Geometry: final body of the model. Coordinates: model frame, mm. A direction names the side the tool comes from. Round coordinates to 2 decimals unless told otherwise and drop trailing zeros. Loops run counter-clockwise (first coordinate to the right, second up) from the corner with the lowest first, then second, coordinate; pieces in that order, holes last. Notation, with made-up numbers: (38, 5.25) -> (75, 5.25) arc R28 ccw to (75, 31.25) -> close; hole circle Ø1 at (37.25, 17.5). An arc over 180 degrees is marked (long way). Answer in a Markdown table with one row per item.
```python
from build123d import *

# Parameters (mm, degrees)
SKETCH1_R           = 2.75
BOSS_EXTRUDE1_DEPTH = 12
SKETCH2_W           = 16
SKETCH2_H           = 46.496113018
CUT_EXTRUDE1_DEPTH  = 229.638147517
SKETCH3_R           = 2.1
CUT_EXTRUDE2_DEPTH  = 229.638147517
CUT_EXTRUDE3_DEPTH  = 229.638147517
FILLET1_R           = 3
FILLET2_R           = 2
SKETCH6_R           = 1.8
CUT_EXTRUDE4_DEPTH  = 229.638147652
CHAMFER1_SIZE       = 1.678199262
CHAMFER1_SIZE_2     = 2


with BuildPart() as part:
    # Sketch1 → Boss-Extrude1 (new body)
    with BuildSketch(Plane(origin=(0, 0, 0), x_dir=(1, 0, 0), z_dir=(0, 1, 0))):
        with BuildLine():
            Line((0, 71.75), (68.4, 71.75))
            Line((68.4, 71.75), (74.4, 82.75))
            Line((74.4, 82.75), (119.4, 82.75))
            Line((119.4, 82.75), (125.4, 71.75))
            Line((125.4, 71.75), (212.8, 71.75))
            Line((212.8, 71.75), (212.8, 43.975))
            Line((212.8, 43.975), (202.281088693, 43.975))
            ThreePointArc((202.281088693, 43.975), (201.490544346, 44.652363805), (200.7, 43.975))
            Line((200.7, 43.975), (200.7, 27.775))
            ThreePointArc((200.7, 27.775), (201.490544346, 27.097636195), (202.281088693, 27.775))
            Line((202.281088693, 27.775), (212.8, 27.775))
            Line((212.8, 27.775), (212.8, 0))
            Line((212.8, 0), (106.4, 0))
            Line((106.4, 0), (0, 0))
            Line((0, 0), (0, 27.775))
            Line((0, 27.775), (10.518911307, 27.775))
            ThreePointArc((10.518911307, 27.775), (11.309455654, 27.097636195), (12.1, 27.775))
            Line((12.1, 27.775), (12.1, 43.975))
            ThreePointArc((12.1, 43.975), (11.309455654, 44.652363805), (10.518911307, 43.975))
            Line((10.518911307, 43.975), (0, 43.975))
            Line((0, 43.975), (0, 71.75))
        make_face()
        with Locations(Location((39, 59.75, 0), (0, 0, 270))):
            Circle(SKETCH1_R, mode=Mode.SUBTRACT)
        with Locations(Location((39, 12, 0), (0, 0, 270))):
            Circle(SKETCH1_R, mode=Mode.SUBTRACT)
        with Locations(Location((173.8, 59.75, 0), (0, 0, 90))):
            Circle(SKETCH1_R, mode=Mode.SUBTRACT)
        with Locations(Location((173.8, 12, 0), (0, 0, 90))):
            Circle(SKETCH1_R, mode=Mode.SUBTRACT)
        with Locations(Location((6, 12, 0), (0, 0, 270))):
            Circle(SKETCH1_R, mode=Mode.SUBTRACT)
        with Locations(Location((6, 59.75, 0), (0, 0, 270))):
            Circle(SKETCH1_R, mode=Mode.SUBTRACT)
        with Locations(Location((206.8, 59.75, 0), (0, 0, 90))):
            Circle(SKETCH1_R, mode=Mode.SUBTRACT)
        with Locations(Location((206.8, 12, 0), (0, 0, 90))):
            Circle(SKETCH1_R, mode=Mode.SUBTRACT)
        with BuildLine():
            Line((32.95, 36.1), (32.95, 19.9))
            ThreePointArc((32.95, 19.9), (33.75, 19.1), (34.55, 19.9))
            Line((34.55, 19.9), (43.45, 19.9))
            ThreePointArc((43.45, 19.9), (44.25, 19.1), (45.05, 19.9))
            Line((45.05, 19.9), (45.05, 36.1))
            ThreePointArc((45.05, 36.1), (44.25, 36.9), (43.45, 36.1))
            Line((43.45, 36.1), (34.55, 36.1))
            ThreePointArc((34.55, 36.1), (33.75, 36.9), (32.95, 36.1))
        make_face(mode=Mode.SUBTRACT)
        with BuildLine():
            Line((179.85, 36.1), (179.85, 19.9))
            ThreePointArc((179.85, 19.9), (179.05, 19.1), (178.25, 19.9))
            Line((178.25, 19.9), (169.35, 19.9))
            ThreePointArc((169.35, 19.9), (168.55, 19.1), (167.75, 19.9))
            Line((167.75, 19.9), (167.75, 36.1))
            ThreePointArc((167.75, 36.1), (168.55, 36.9), (169.35, 36.1))
            Line((169.35, 36.1), (178.25, 36.1))
            ThreePointArc((178.25, 36.1), (179.05, 36.9), (179.85, 36.1))
        make_face(mode=Mode.SUBTRACT)
    extrude(amount=BOSS_EXTRUDE1_DEPTH)

    # Sketch2 → Cut-Extrude1 (cut, through all)
    with BuildSketch(Plane(origin=(0, 12, 0), x_dir=(1, 0, 0), z_dir=(0, 1, 0))):
        with Locations((58.05, 61.998056509)):
            Rectangle(SKETCH2_W, SKETCH2_H)
    extrude(amount=-CUT_EXTRUDE1_DEPTH, mode=Mode.SUBTRACT)

    # Sketch3 → Cut-Extrude2 (cut, through all)
    with BuildSketch(Plane(origin=(0, 12, 0), x_dir=(1, 0, 0), z_dir=(0, 1, 0))):
        with Locations(Location((78.05, 78.75, 0), (0, 0, 270))):
            Circle(SKETCH3_R)
        with Locations(Location((78.05, 46.75, 0), (0, 0, 270))):
            Circle(SKETCH3_R)
        with Locations(Location((116.05, 78.75, 0), (0, 0, 270))):
            Circle(SKETCH3_R)
        with Locations(Location((116.05, 46.75, 0), (0, 0, 270))):
            Circle(SKETCH3_R)
    extrude(amount=-CUT_EXTRUDE2_DEPTH, mode=Mode.SUBTRACT)

    # Sketch5 → Cut-Extrude3 (cut, through all)
    with BuildSketch(Plane(origin=(0, 12, 0), x_dir=(1, 0, 0), z_dir=(0, 1, 0))):
        with BuildLine():
            Line((98.782125318, 39), (82.518680026, 39))
            ThreePointArc((82.518680026, 39), (80.72736119, 38.668102058), (79.173856368, 37.716470731))
            Line((79.173856368, 37.716470731), (65.279045214, 25.211140692))
            ThreePointArc((65.279045214, 25.211140692), (64.056368555, 23.528862886), (63.623868872, 21.494669961))
            Line((63.623868872, 21.494669961), (63.623868872, 17))
            ThreePointArc((63.623868872, 17), (65.088334966, 13.464466094), (68.623868872, 12))
            Line((68.623868872, 12), (74.681319974, 12))
            ThreePointArc((74.681319974, 12), (76.47263881, 12.331897942), (78.026143632, 13.283529269))
            Line((78.026143632, 13.283529269), (100.789019513, 33.770117561))
            ThreePointArc((100.789019513, 33.770117561), (101.582986553, 37.074791302), (98.782125318, 39))
        make_face()
        with BuildLine():
            Line((115.851322474, 37.77611222), (94.075922745, 17.179491723))
            ThreePointArc((94.075922745, 17.179491723), (93.350095678, 13.890602679), (96.13743089, 12))
            Line((96.13743089, 12), (141.06256911, 12))
            ThreePointArc((141.06256911, 12), (143.849904322, 13.890602679), (143.124077255, 17.179491723))
            Line((143.124077255, 17.179491723), (121.348677526, 37.77611222))
            ThreePointArc((121.348677526, 37.77611222), (118.6, 38.870123257), (115.851322474, 37.77611222))
        make_face()
        with BuildLine():
            Line((138.417874682, 39), (156.6, 39))
            ThreePointArc((156.6, 39), (159.428427125, 37.828427125), (160.6, 35))
            Line((160.6, 35), (160.6, 18.736087214))
            ThreePointArc((160.6, 18.736087214), (158.820515755, 15.995587024), (155.593105805, 16.506204775))
            Line((155.593105805, 16.506204775), (136.410980487, 33.770117561))
            ThreePointArc((136.410980487, 33.770117561), (135.617013447, 37.074791302), (138.417874682, 39))
        make_face()
        with BuildLine():
            Line((86.05, 73.75), (108.05, 73.75))
            ThreePointArc((108.05, 73.75), (110.878427125, 72.578427125), (112.05, 69.75))
            Line((112.05, 69.75), (112.05, 54.75))
            ThreePointArc((112.05, 54.75), (110.878427125, 51.921572875), (108.05, 50.75))
            Line((108.05, 50.75), (86.05, 50.75))
            ThreePointArc((86.05, 50.75), (83.221572875, 51.921572875), (82.05, 54.75))
            Line((82.05, 54.75), (82.05, 69.75))
            ThreePointArc((82.05, 69.75), (83.221572875, 72.578427125), (86.05, 73.75))
        make_face()
        with BuildLine():
            Line((129.75, 61.75), (157.75, 61.75))
            ThreePointArc((157.75, 61.75), (160.578427125, 60.578427125), (161.75, 57.75))
            Line((161.75, 57.75), (161.75, 47.75))
            ThreePointArc((161.75, 47.75), (160.578427125, 44.921572875), (157.75, 43.75))
            Line((157.75, 43.75), (129.75, 43.75))
            ThreePointArc((129.75, 43.75), (126.921572875, 44.921572875), (125.75, 47.75))
            Line((125.75, 47.75), (125.75, 57.75))
            ThreePointArc((125.75, 57.75), (126.921572875, 60.578427125), (129.75, 61.75))
        make_face()
    extrude(amount=-CUT_EXTRUDE3_DEPTH, mode=Mode.SUBTRACT)

    # Fillet1
    fillet1_edges = [part.edges().sort_by_distance(p)[0] for p in [
        (50.05, 6, -38.75),
        (66.05, 6, -38.75),
        (68.4, 6, -71.75),
        (125.4, 6, -71.75),
    ]]
    fillet(fillet1_edges, radius=FILLET1_R)

    # Fillet2
    fillet2_edges = [part.edges().sort_by_distance(p)[0] for p in [
        (212.8, 6, -71.75),
        (119.4, 6, -82.75),
        (74.4, 6, -82.75),
        (50.05, 6, -71.75),
        (66.05, 6, -71.75),
        (0, 6, -71.75),
        (212.8, 6, 0),
        (0, 6, 0),
    ]]
    fillet(fillet2_edges, radius=FILLET2_R)

    # Sketch6 → Cut-Extrude4 (cut, through all)
    with BuildSketch(Plane(origin=(0, 12, 0), x_dir=(1, 0, 0), z_dir=(0, 1, 0))):
        with Locations(Location((186.8, 45, 0), (0, 0, 270))):
            Circle(SKETCH6_R)
        with Locations(Location((186.8, 15, 0), (0, 0, 270))):
            Circle(SKETCH6_R)
        with Locations(Location((23.8, 45, 0), (0, 0, 90))):
            Circle(SKETCH6_R)
        with Locations(Location((23.8, 15, 0), (0, 0, 90))):
            Circle(SKETCH6_R)
    extrude(amount=-CUT_EXTRUDE4_DEPTH, mode=Mode.SUBTRACT)

    # Chamfer1
    # the kernel refuses this chamfer: 2, 1.678199262 mm, written as the material it takes off along each edge
    with BuildSketch(Plane(origin=(78.05, 12, -46.75), x_dir=(0, 0, 1), z_dir=(-1, 0, 0))) as chamfer1_piece_1:
        Polygon((2.1, -CHAMFER1_SIZE), (2.1 + CHAMFER1_SIZE_2, 0), (2.1, 0), align=None)
    revolve(axis=Axis((78.05, 12, -46.75), (0, 1, 0)), mode=Mode.SUBTRACT)
    with BuildSketch(Plane(origin=(116.05, 12, -78.75), x_dir=(0, 0, 1), z_dir=(-1, 0, 0))) as chamfer1_piece_2:
        Polygon((2.1, -CHAMFER1_SIZE), (2.1 + CHAMFER1_SIZE_2, 0), (2.1, 0), align=None)
    revolve(axis=Axis((116.05, 12, -78.75), (0, 1, 0)), mode=Mode.SUBTRACT)
    with BuildSketch(Plane(origin=(116.05, 12, -46.75), x_dir=(0, 0, 1), z_dir=(-1, 0, 0))) as chamfer1_piece_3:
        Polygon((2.1, -CHAMFER1_SIZE), (2.1 + CHAMFER1_SIZE_2, 0), (2.1, 0), align=None)
    revolve(axis=Axis((116.05, 12, -46.75), (0, 1, 0)), mode=Mode.SUBTRACT)
    with BuildSketch(Plane(origin=(78.05, 12, -78.75), x_dir=(0, 0, 1), z_dir=(-1, 0, 0))) as chamfer1_piece_4:
        Polygon((2.1, -CHAMFER1_SIZE), (2.1 + CHAMFER1_SIZE_2, 0), (2.1, 0), align=None)
    revolve(axis=Axis((78.05, 12, -78.75), (0, 1, 0)), mode=Mode.SUBTRACT)


solid = part.part
```
Item 1: Set-up query: faces 1 (the conical face through (80.26, 10.43, -79.04)), 2 (the flat face through (207, 6, -27.775)), 3 (the flat face through (125.75, 6, -53)), 4 (the flat face through (108, 0, -33)), 5 (the flat face through (25, 6, -71.75)). Return all of +Z, -Z, +X, -X, +Y, -Y with unobstructed straight access to the full face (end or side cutting, diameter ignored); none if empty.
Ans:
| item | result |
|---|---|
| face 1 | +Y |
| face 2 | +X, +Y, -Y |
| face 3 | +Y, -Y |
| face 4 | +Z, -Z, +X, -X, -Y |
| face 5 | -Z, -X, +Y, -Y |
Item 2: Ray query, L1, parallel to Z at x = 173.8, y = 8.75; L2, parallel to Z at x = 186.5, y = 3; L3, parallel to Z at x = 158, y = 7.25. Return the intervals inside material, ascending.
Ans:
| item | result |
|---|---|
| L1 | -71.75 to -62.5, -57 to -36.1, -19.9 to -14.75, -9.25 to 0 |
| L2 | -71.75 to -46.77, -43.23 to -16.77, -13.23 to 0 |
| L3 | -71.75 to -61.74, -43.76 to -38.75, -15.76 to 0 |
Item 3: First-contact query: P1, Ø2.5, axis at x = 172.5, y = 6, coming from the -Z side; P2, Ø3.5, axis at x = 78.05, z = -78.75, coming from the -Y side; P3, Ø3.5, axis at y = 5.5, z = -31.5, coming from the -X side. Flat tips, straight axial feed; report the tip coordinate or a pass-through.
Ans:
| item | result |
|---|---|
| P1 | z = -71.75 |
| P2 | through |
| P3 | x = 12.1 |
Item 4: Section query B-B, the plane y = 4.5. State how many separate pieces and enclosed holes the cut face has, and give its area (3 significant figures).
Ans:
| item | result |
|---|---|
| separate pieces | 1 |
| enclosed holes | 23 |
| area | 11,100 mm2 |
Item 5: Section query A-A, the plane x = 173.8. Output: boundary loops of the cut face in (y, z).
Ans:
| item | result |
|---|---|
| outline | (0, -71.75) -> (12, -71.75) -> (12, -62.5) -> (0, -62.5) -> close; (0, -57) -> (12, -57) -> (12, -36.1) -> (0, -36.1) -> close; (0, -19.9) -> (12, -19.9) -> (12, -14.75) -> (0, -14.75) -> close; (0, -9.25) -> (12, -9.25) -> (12, 0) -> (0, 0) -> close |
Item 6: Mould query, pull axis X, two halves, no side actions, for faces 6 (the flat face through (71.51, 5.92, -77.45)), 7 (the flat face through (5, 6, -27.775)), 8 (the flat face through (144, 6, -61.75)). Classes: released by +X, released by -X, zero draft, split by the parting line, or undercut.
Ans:
| item | result |
|---|---|
| face 6 | released by -X |
| face 7 | zero draft |
| face 8 | undercut |
